Source: CAD feature listing. Evaluate the final solid. Frame: model axes, mm. Face numbers are marked on the shaded views. A direction names the side the tool comes from. Coordinates: 2 decimals unless noted, no trailing zeros. Loops run counter-clockwise (first coordinate to the right, second up) from the corner with the lowest first, then second, coordinate; pieces in that order, holes last.
Item 1: Section query D-D, the plane x = 8. Return the cut outline in (y, z), then the cut area to 3 significant figures.
Item 2: Section query C-C, the plane z = -2.5. Return the cut outline in (x, y).
Item 3: Reachability of the marked faces 5, 6 and 7 from +Z, -Z, +X, -X, +Y, -Y: full face, straight path, thin tool, end or side. Return the list, or none.
Item 4: Section query B-B, the plane y = 36.5. State how many separate pieces and enclosed holes the cut face has, then the cut area to 3 significant figures.
Item 5: Section query A-A, the plane x = -5. Return the cut outline in (y, z) (3 decimals), then the cut area to 3 significant figures.
Item 6: Line query: probe 1 along Y at (x, z) = (8, -2.25); probe 2 along X at (y, z) = (36.5, -5.5); probe 3 along Y at (x, z) = (24, 10). Output: solid intervals per line, ascending.
Item 7: Pull-direction query (Y, two-part tool) for the marked faces 1, 2, 3 and 4; classes: +Y half, -Y half, draft (parallel to the pull), parting line (faces both ways), or undercut.
Item 8: Pin query (flat end, axial travel): pin 1 Ø21.5 at (x, y) = (8, 36.5) entering from +Z; pin 2 Ø2 at (y, z) = (46.5, 7) entering from -X; pin 3 Ø5 at (x, y) = (0, 36.5) entering from +Z; pin 4 Ø5 at (x, y) = (-5, 49) entering from +Z. Return the tip coordinate at first contact, or that it passes through.
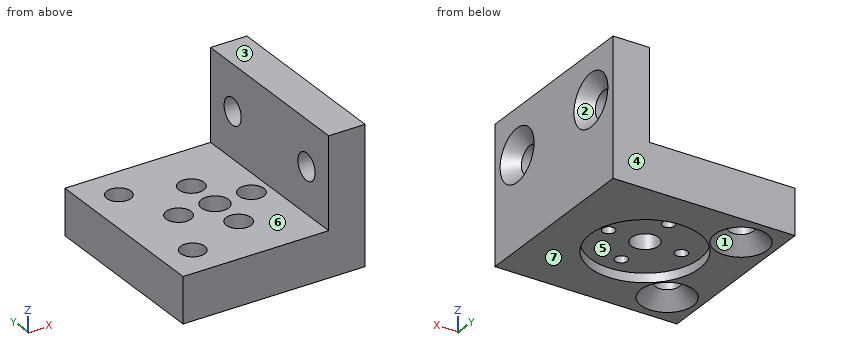
Solid Edge part; units mm, degrees
sketch "Sketch1" plane through (0, 0, 0) normal (0, 0, -1) x (-1, 0, 0)
  line L0 (12, 56.5) -> (12, 16.5)
  line L1 (-28, 16.5) -> (12, 16.5)
  line L2 (-28, 56.5) -> (-28, 16.5)
  line L3 (12, 56.5) -> (-28, 56.5)
  dimension "D1" = 12
  dimension "D2" = 28
extrude "Protrusion1" add sketch "Sketch1" along normal blind 10
sketch "Sketch2" plane through (8, 16.5, -5) normal (0, -1, 0) x (1, 0, 0)
  line L0 (12, 25) -> (12, 5)
  line L1 (12, 5) -> (20, 5)
  line L2 (20, 5) -> (20, 25)
  line L3 (20, 25) -> (12, 25)
  dimension "D1" = 20
  dimension "D2" = 12
extrude "Protrusion2" add sketch "Sketch2" against normal up to vertex (40 mm away)
sketch "Sketch3" plane through (8, 36.5, -10) normal (0, 0, -1) x (1, 0, 0)
  circle A0 centre (0, 0) radius 12
extrude "VaciadoExtruido_1" cut sketch "Sketch3" against normal blind 2
hole "Agujero_1" at (-5, 49, -10) direction (0, 0, 1) diameter 5.3 end up to next countersink diameter 11.47 countersink angle 90
hole "Hole1" at (-5, 24, -10) direction (0, 0, 1) diameter 5.3 end up to next countersink diameter 11.47 countersink angle 90
hole "Agujero_3" at (28, 49, 10) direction (-1, 0, 0) diameter 5.8 end up to next countersink diameter 11.47 countersink angle 90
hole "Hole2" at (28, 24, 10) direction (-1, 0, 0) diameter 5.8 end up to next countersink diameter 11.47 countersink angle 90
hole "Agujero_6" at (16, 36.5, 0) direction (0, 0, -1) diameter 2.7 end up to next counterbore diameter 5.5 counterbore depth 5
hole "Hole3" at (8, 28.5, 0) direction (0, 0, -1) diameter 2.7 end up to next counterbore diameter 5.5 counterbore depth 5
hole "Hole4" at (8, 44.5, 0) direction (0, 0, -1) diameter 2.7 end up to next counterbore diameter 5.5 counterbore depth 5
hole "Hole5" at (0, 36.5, 0) direction (0, 0, -1) diameter 2.7 end up to next counterbore diameter 5.5 counterbore depth 5
sketch "Sketch4" plane through (4, 36.5, 0) normal (0, 0, 1) x (0, 1, 0)
  circle A0 centre (0, -4) radius 3
extrude "Cutout1" cut sketch "Sketch4" against normal up to next
properties part number "1976-1500-007" material "Aluminio, 7075-T6"
Verdict:
1. outline: (16.5, -10) - (24.5, -10) - (24.5, -8) - (27.15, -8) - (27.15, -5) - (25.75, -5) - (25.75, 0) - (16.5, 0) - close; (29.85, -8) - (33.5, -8) - (33.5, 0) - (31.25, 0) - (31.25, -5) - (29.85, -5) - close; (39.5, -8) - (43.15, -8) - (43.15, -5) - (41.75, -5) - (41.75, 0) - (39.5, 0) - close; (45.85, -8) - (48.5, -8) - (48.5, -10) - (56.5, -10) - (56.5, 0) - (47.25, 0) - (47.25, -5) - (45.85, -5) - close
1. area: 233 mm2
2. outline: (-12, 16.5) - (28, 16.5) - (28, 56.5) - (-12, 56.5) - close; hole circle Ø5.3 at (-5, 24); hole circle Ø5.3 at (-5, 49); hole circle Ø5.5 at (0, 36.5); hole circle Ø6 at (8, 36.5); hole circle Ø5.5 at (8, 28.5); hole circle Ø5.5 at (8, 44.5); hole circle Ø5.5 at (16, 36.5)
3. face 5: -Z
3. face 6: +Z, -X, +Y, -Y
3. face 7: -Z, +X, -X, +Y, -Y
4. separate pieces: 4
4. enclosed holes: 0
4. area: 393 mm2
5. outline: (16.5, -10) - (18.265, -10) - (21.35, -6.915) - (21.35, 0) - (16.5, 0) - close; (26.65, -6.915) - (29.735, -10) - (43.265, -10) - (46.35, -6.915) - (46.35, 0) - (26.65, 0) - close; (51.65, -6.915) - (54.735, -10) - (56.5, -10) - (56.5, 0) - (51.65, 0) - close
5. area: 275 mm2
6. probe 1: y = 16.5 to 25.75, 31.25 to 33.5, 39.5 to 41.75, 47.25 to 56.5
6. probe 2: x = -12 to -1.35, 1.35 to 5, 11 to 14.65, 17.35 to 28
6. probe 3: y = 16.5 to 21.1, 26.9 to 46.1, 51.9 to 56.5
7. face 1: undercut
7. face 2: undercut
7. face 3: draft
7. face 4: +Y half
8. pin 1: stops at z = 0
8. pin 2: stops at x = 20
8. pin 3: stops at z = -5
8. pin 4: passes through
